The listing builds one solid part. Answer for the finished solid, in the listing's coordinates (mm). Face numbers are marked on the shaded views. A direction names the side the tool comes from. Give positions to 0.01 mm unless a question says otherwise; leave off trailing zeros. Answer as a JSON object with one key per item and string values.
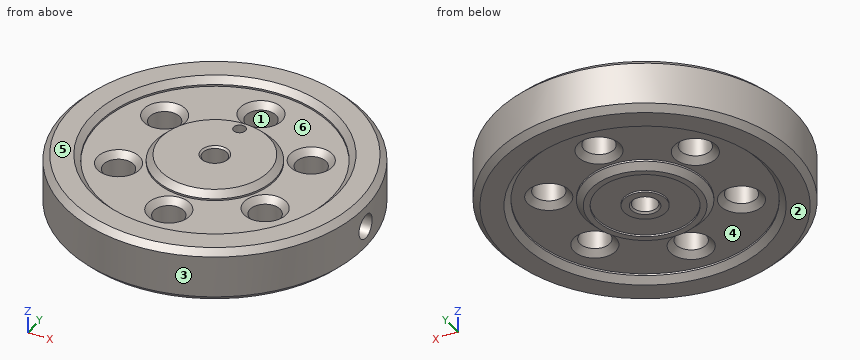
```python
from build123d import *

# Parameters (mm, degrees)
SKETCH_1_R               = 25
EXTRUDE_1_DEPTH          = 4.5
SKETCH_2_R               = 2
CUT_EXTRUDE_1_DEPTH      = 37.482872694
CHAMFER_1_SIZE           = 1
SKETCH_3_R               = 19.5
SKETCH_3_R_2             = 10
CUT_EXTRUDE_2_DEPTH      = 1.3
CHAMFER_2_SIZE           = 1
CHAMFER_3_SIZE           = 1
SKETCH_4_R               = 1
CUT_EXTRUDE_3_DEPTH      = 2
CHAMFER_4_SIZE           = 0.3
CHAMFER_5_SIZE           = 1
SKETCH_5_R               = 8
SKETCH_5_R_2             = 3.5
CUT_EXTRUDE_4_DEPTH      = 0.3
SKETCH_6_R               = 2.5
CUT_EXTRUDE_5_DEPTH      = 37.184112536
CHAMFER_6_SIZE           = 1
CUT_EXTRUDE_START        = 10
SKETCH_7_R               = 2
CUT_EXTRUDE_6_DEPTH      = 20
CUT_EXTRUDE_7_REACH      = 45.246
CUT_EXTRUDE_7_END_RADIUS = 2
SKETCH_8_R               = 1.5


with BuildPart() as part:
    # 草图1 → 凸台-拉伸1 (new, symmetric)
    with BuildSketch(Plane.XY):
        Circle(SKETCH_1_R)
    extrude(amount=EXTRUDE_1_DEPTH, both=True)

    # 草图2 → 切除-拉伸1 (cut, through all)
    with BuildSketch(Plane.XY.offset(4.5)):
        Circle(SKETCH_2_R)
    extrude(amount=-CUT_EXTRUDE_1_DEPTH, mode=Mode.SUBTRACT)

    # 倒角1
    chamfer_1_edges = [part.edges().sort_by_distance(p)[0] for p in [
        (-25, 0, -4.5),
        (-25, 0, 4.5),
    ]]
    chamfer(chamfer_1_edges, length=CHAMFER_1_SIZE)

    # 草图3 → 切除-拉伸2 (cut)
    with BuildSketch(Plane.XY.offset(4.5)):
        Circle(SKETCH_3_R)
        Circle(SKETCH_3_R_2, mode=Mode.SUBTRACT)
    cut_extrude_2 = extrude(amount=-CUT_EXTRUDE_2_DEPTH, mode=Mode.SUBTRACT)

    # 倒角2
    chamfer_2_edges = [part.edges().sort_by_distance(p)[0] for p in [
        (-19.5, 0, 4.5),
    ]]
    chamfer(chamfer_2_edges, length=CHAMFER_2_SIZE)

    # 倒角3
    chamfer_3_edges = [part.edges().sort_by_distance(p)[0] for p in [
        (-10, 0, 4.5),
    ]]
    chamfer(chamfer_3_edges, length=CHAMFER_3_SIZE)

    # 草图4 → 切除-拉伸3 (cut)
    with BuildSketch(Plane.XY.offset(4.5)):
        with Locations((0, 7.5)):
            Circle(SKETCH_4_R)
    extrude(amount=-CUT_EXTRUDE_3_DEPTH, mode=Mode.SUBTRACT)

    # 倒角4
    chamfer_4_edges = [part.edges().sort_by_distance(p)[0] for p in [
        (-2, 0, -4.5),
        (-2, 0, 4.5),
    ]]
    chamfer(chamfer_4_edges, length=CHAMFER_4_SIZE)

    # 镜向3: 切除-拉伸2 across plane
    add(cut_extrude_2.mirror(Plane.XY), mode=Mode.SUBTRACT)

    # 倒角5
    chamfer_5_edges = [part.edges().sort_by_distance(p)[0] for p in [
        (-10, 0, -4.5),
        (-19.5, 0, -4.5),
    ]]
    chamfer(chamfer_5_edges, length=CHAMFER_5_SIZE)

    # 草图5 → 切除-拉伸4 (cut)
    with BuildSketch(Plane(origin=(0, 0, -4.5), x_dir=(-1, 0, 0), z_dir=(0, 0, -1))):
        Circle(SKETCH_5_R)
        Circle(SKETCH_5_R_2, mode=Mode.SUBTRACT)
    extrude(amount=-CUT_EXTRUDE_4_DEPTH, mode=Mode.SUBTRACT)

    # 草图6 → 切除-拉伸5 (cut, through all)
    with BuildSketch(Plane.XY.offset(3.2)):
        with Locations((0, 14)):
            Circle(SKETCH_6_R)
        with Locations((12.124355653, 7)):
            Circle(SKETCH_6_R)
        with Locations((12.124355653, -7)):
            Circle(SKETCH_6_R)
        with Locations((0, -14)):
            Circle(SKETCH_6_R)
        with Locations((-12.124355653, -7)):
            Circle(SKETCH_6_R)
        with Locations((-12.124355653, 7)):
            Circle(SKETCH_6_R)
    extrude(amount=-CUT_EXTRUDE_5_DEPTH, mode=Mode.SUBTRACT)

    # 倒角6
    chamfer_6_edges = [part.edges().sort_by_distance(p)[0] for p in [
        (-2.5, 14, -3.2),
        (-2.5, 14, 3.2),
        (-14.624355653, 7, -3.2),
        (-14.624355653, 7, 3.2),
        (-14.624355653, -7, -3.2),
        (-14.624355653, -7, 3.2),
        (-2.5, -14, -3.2),
        (-2.5, -14, 3.2),
        (9.624355653, -7, -3.2),
        (9.624355653, -7, 3.2),
        (9.624355653, 7, -3.2),
        (9.624355653, 7, 3.2),
    ]]
    chamfer(chamfer_6_edges, length=CHAMFER_6_SIZE)

    # 草图7 → 切除-拉伸6 (cut)
    with BuildSketch(Plane(origin=(0, 0, 0), x_dir=(0, 0, -1), z_dir=(1, 0, 0)).offset(CUT_EXTRUDE_START)):
        Circle(SKETCH_7_R)
    extrude(amount=CUT_EXTRUDE_6_DEPTH, mode=Mode.SUBTRACT)

    # 切除-拉伸7: up to this cylinder (the profile starts outside it)
    cut_extrude_7_end = Plane(origin=(0, 0, 0), z_dir=(0, 0, 1)) * Cylinder(CUT_EXTRUDE_7_END_RADIUS, 95.492, mode=Mode.PRIVATE)
    # 草图8 → 切除-拉伸7 (cut, up to the surface)
    with BuildSketch(Plane(origin=(10, 0, 0), x_dir=(0, 0, -1), z_dir=(1, 0, 0)), mode=Mode.PRIVATE) as cut_extrude_7_sk1:
        Circle(SKETCH_8_R)
    cut_extrude_7_tool1 = extrude(cut_extrude_7_sk1.sketch, amount=-CUT_EXTRUDE_7_REACH, mode=Mode.PRIVATE) - cut_extrude_7_end
    add(cut_extrude_7_tool1.solids().sort_by_distance((10, 0, 0))[0], mode=Mode.SUBTRACT)


solid = part.part
```
1. For the marked faces 4, 5 and 6, determine the directions among +Z, -Z, +X, -X, +Y, -Y from which every point of the face is accessible in a straight line to the end or side of a thin tool.
Verdict:
{"face 4": "-Z", "face 5": "+Z, +X, -X, +Y, -Y", "face 6": "+Z"}
2. The mould has two halves that part along Y. Classify the marked faces 1, 2 and 3: released by +Y, released by -Y, zero draft, split by the parting line, or undercut.
Verdict:
{"face 1": "undercut", "face 2": "zero draft", "face 3": "split by the parting line"}
3. A cutting plane is placed at A-A, the plane y = 0. Count the separate pieces of the cut face and the enclosed holes in it, plus the area to 3 significant figures.
Verdict:
{"separate pieces": "3", "enclosed holes": "0", "area": "272 mm2"}
4. Flat-ended cylindrical pins translate along their axes: pin 1 (4 mm diameter, centred on y = 5.5, z = -1, fed in from -X); pin 2 (5 mm diameter, centred on y = -7, z = 2, fed in from -X); pin 3 (2 mm diameter, centred on y = -0.5, z = -1, fed in from +X). Find the tip coordinate at first contact, or state that the pin passes through.
Verdict:
{"pin 1": "stops at x = -24.75", "pin 2": "stops at x = -24.59", "pin 3": "stops at x = 25"}
5. Consider line 1 along X through (y, z) = (5.5, 4.25); line 2 along Y through (x, z) = (-1.5, -3.5); line 3 along X through (y, z) = (-10.5, 3.5). Determine where each line is inside the solid, lowest interval first.
Verdict:
{"line 1": "x = -23.62 to -19.49, -7.44 to 7.44, 19.49 to 23.62", "line 2": "y = -24.95 to -19.44, -9.89 to -1.32, 1.32 to 9.89, 19.44 to 24.95", "line 3": "x = -22.69 to -16.43, 16.43 to 22.69"}
